Read the model definition and answer for the solid it produces. Units are mm, in the model's axes. A direction names the side the tool comes from. Coordinates: 2 decimals unless noted, no trailing zeros. Loops run counter-clockwise (first coordinate to the right, second up) from the corner with the lowest first, then second, coordinate; pieces in that order, holes last. Notation, with made-up numbers: (26.25, 22) -> (75.25, 22) arc R26 cw to (75.25, 45) -> close; hole circle Ø6 at (-17.75, 0). An arc over 180 degrees is marked (long way). Answer as a JSON object with one key per item and string values. Group by question number.
1) Section A-A, the plane y = -42 is taken. Give the vertices of the cut face in (x, z).
2) Flat-ended cylindrical pins translate along their axes: P1, Ø0.9, axis at x = -29, z = 55.5, coming from the +Y side; P2, Ø7, axis at y = 22, z = -91.5, coming from the -X side; P3, Ø5, axis at x = -17.5, z = -80, coming from the -Y side; P4, Ø3.5, axis at x = -28.5, y = 14, coming from the +Z side. Find the tip coordinate at first contact, or state that the pin passes through.
3) Consider probe 1 along Y at (x, z) = (-28.75, -76.5); probe 2 along Z at (x, y) = (25, -5); probe 3 along Y at (x, z) = (16, 72). Determine where each line is inside the solid, lowest interval first. Write a range as [from, to].
4) Which of the six approach directions +Z, -Z, +X, -X, +Y, -Y give full straight-line access (tool end or side, diameter ignored) to faces 4 (the face through (27.2, 6.6, -110)), 5 (the face through (25.98, -23.707, -115.521)), 6 (the face through (-28.479, 22.121, -73.753))?
5) Section C-C, the plane x = 2.5 is taken. Give the vertices of the cut face in (y, z).
6) Determine the mould class of faces 1 (the face through (1.08, 1.48, 99.88)), 2 (the face through (-29, 28, -96)), 3 (the face through (-23, -1, -113)) for opening direction Z: released by +Z, released by -Z, zero draft, split by the parting line, or undercut.
7) Section D-D, the plane y = -68 is taken. Give the vertices of the cut face in (x, z), plus the area to 3 significant figures.
8) Section B-B, the plane z = 51 is taken. Give the vertices of the cut face in (x, y).
from build123d import *

# Parameters (mm, degrees)
ODGI_CIE_BAZOWE1_DEPTH           = 110
ODGI_CIE_START                   = -40
ODGI_CIE_KRAW_DZI1_OUTLINE_W     = 73
ODGI_CIE_KRAW_DZI1_OUTLINE_H     = 3
ODGI_CIE_KRAW_DZI1_DEPTH         = 80
ODGI_CIE_START_2                 = -23
ODGI_CIE_KRAW_DZI1_2_DEPTH       = 46
WYTNIJ_WYCI_GNI_CIE1_REACH       = 245.019
OTW_R_POD_RUB_M81_D              = 10
OTW_R_POD_RUB_M81_DEPTH          = 10
OTW_R_POD_RUB_M81_TIP            = 3.004303095
SZKIC19_W                        = 25
SZKIC19_H                        = 15
WYTNIJ_WYCI_GNI_CIE2_DEPTH       = 10
ZAOKR_GLENIE1_R                  = 2
WYTNIJ_WYCI_GNI_CIE3_REACH       = 245.019
SZKIC20_R                        = 6.5
WYTNIJ_WYCI_GNI_CIE4_DEPTH       = 157.582246759
ZAOKR_GLENIE2_R                  = 1
SZYK_LINIOWY1_COUNT              = 3
SZYK_LINIOWY1_PITCH              = 70
ZAOKR_GLENIE2_OF_SZYK_LINIOWY1_R = 1
SZKIC22_R                        = 6
WYTNIJ_WYCI_GNI_CIE5_DEPTH       = 244.018517813
ZAOKR_GLENIE3_R                  = 12
SZKIC23_W                        = 30
SZKIC23_H                        = 12
WYPUST2_DEPTH                    = 3
SFAZOWANIE1_SIZE                 = 5
OTW_R_POD_RUB_M52_D              = 5.5


# Read off the part's stored shape, not the designer's step: Odgięcie krawędzi1
# Sheet-metal steps are written as plain solids
with BuildPart() as part:
    # Szkic1 → Odgięcie bazowe1 (new, symmetric)
    with BuildSketch(Plane.XY):
        with BuildLine():
            Line((-30, 18), (-30, 7))
            ThreePointArc((-30, 7), (-27.949747468, 2.050252532), (-23, 0))
            Line((-23, 0), (23, 0))
            ThreePointArc((23, 0), (27.949747468, 2.050252532), (30, 7))
            Line((30, 7), (30, 18))
            Line((30, 18), (27, 18))
            Line((27, 18), (27, 7))
            ThreePointArc((27, 7), (25.828427125, 4.171572875), (23, 3))
            Line((23, 3), (-23, 3))
            ThreePointArc((-23, 3), (-25.828427125, 4.171572875), (-27, 7))
            Line((-27, 7), (-27, 18))
            Line((-27, 18), (-30, 18))
        make_face()
    extrude(amount=ODGI_CIE_BAZOWE1_DEPTH, both=True)



with BuildPart() as body_2:
    # Odgięcie krawędzi1 outline → Odgięcie krawędzi1 (new body)
    with BuildSketch(Plane.YZ.offset(ODGI_CIE_START)):
        with Locations((-40.5, -115.5)):
            Rectangle(ODGI_CIE_KRAW_DZI1_OUTLINE_W, ODGI_CIE_KRAW_DZI1_OUTLINE_H)
    extrude(amount=ODGI_CIE_KRAW_DZI1_DEPTH)


with BuildPart() as part_1:
    add(part.part)

    add(body_2.part)  # Odgi_cie kraw_dzi1 2 merges body 2
    # Odgi_cie kraw_dzi1 2 outline → Odgi_cie kraw_dzi1 2 (add)
    with BuildSketch(Plane.YZ.offset(ODGI_CIE_START_2)):
        with BuildLine():
            Line((-4, -114), (-4, -117))
            ThreePointArc((-4, -117), (0.949747468, -114.949747468), (3, -110))
            Line((3, -110), (0, -110))
            ThreePointArc((0, -110), (-1.171572875, -112.828427125), (-4, -114))
        make_face()
    extrude(amount=ODGI_CIE_KRAW_DZI1_2_DEPTH)

    # Szkic9 → Wytnij-wyciągnięcie1 (cut, up to next)
    with BuildSketch(Plane(origin=(0, 0, -117), x_dir=(-1, 0, 0), z_dir=(0, 0, -1)), mode=Mode.PRIVATE) as wytnij_wyci_gni_cie1_sk1:
        with BuildLine():
            Line((-30.018425021, -20.879449696), (-21.826904579, -26.61521406))
            ThreePointArc((-21.826904579, -26.61521406), (-21.151571657, -30.445217382), (-24.981574979, -31.120550304))
            Line((-24.981574979, -31.120550304), (-33.173095421, -25.38478594))
            ThreePointArc((-33.173095421, -25.38478594), (-33.848428343, -21.554782618), (-30.018425021, -20.879449696))
        make_face()
    wytnij_wyci_gni_cie1_tool1 = extrude(wytnij_wyci_gni_cie1_sk1.sketch, amount=-WYTNIJ_WYCI_GNI_CIE1_REACH, mode=Mode.PRIVATE) & part_1.part
    # Szkic9 → Wytnij-wyciągnięcie1 (cut, up to next)
    with BuildSketch(Plane(origin=(0, 0, -117), x_dir=(-1, 0, 0), z_dir=(0, 0, -1)), mode=Mode.PRIVATE) as wytnij_wyci_gni_cie1_sk2:
        with BuildLine():
            Line((30.018425021, -20.879449696), (21.826904579, -26.61521406))
            ThreePointArc((21.826904579, -26.61521406), (21.151571657, -30.445217382), (24.981574979, -31.120550304))
            Line((24.981574979, -31.120550304), (33.173095421, -25.38478594))
            ThreePointArc((33.173095421, -25.38478594), (33.848428343, -21.554782618), (30.018425021, -20.879449696))
        make_face()
    wytnij_wyci_gni_cie1_tool2 = extrude(wytnij_wyci_gni_cie1_sk2.sketch, amount=-WYTNIJ_WYCI_GNI_CIE1_REACH, mode=Mode.PRIVATE) & part_1.part
    # Szkic9 → Wytnij-wyciągnięcie1 (cut, up to next)
    with BuildSketch(Plane(origin=(0, 0, -117), x_dir=(-1, 0, 0), z_dir=(0, 0, -1)), mode=Mode.PRIVATE) as wytnij_wyci_gni_cie1_sk3:
        with BuildLine():
            Line((-30.018425021, -63.120550304), (-21.826904579, -57.38478594))
            ThreePointArc((-21.826904579, -57.38478594), (-21.151571657, -53.554782618), (-24.981574979, -52.879449696))
            Line((-24.981574979, -52.879449696), (-33.173095421, -58.61521406))
            ThreePointArc((-33.173095421, -58.61521406), (-33.848428343, -62.445217382), (-30.018425021, -63.120550304))
        make_face()
    wytnij_wyci_gni_cie1_tool3 = extrude(wytnij_wyci_gni_cie1_sk3.sketch, amount=-WYTNIJ_WYCI_GNI_CIE1_REACH, mode=Mode.PRIVATE) & part_1.part
    # Szkic9 → Wytnij-wyciągnięcie1 (cut, up to next)
    with BuildSketch(Plane(origin=(0, 0, -117), x_dir=(-1, 0, 0), z_dir=(0, 0, -1)), mode=Mode.PRIVATE) as wytnij_wyci_gni_cie1_sk4:
        with BuildLine():
            Line((30.018425021, -63.120550304), (21.826904579, -57.38478594))
            ThreePointArc((21.826904579, -57.38478594), (21.151571657, -53.554782618), (24.981574979, -52.879449696))
            Line((24.981574979, -52.879449696), (33.173095421, -58.61521406))
            ThreePointArc((33.173095421, -58.61521406), (33.848428343, -62.445217382), (30.018425021, -63.120550304))
        make_face()
    wytnij_wyci_gni_cie1_tool4 = extrude(wytnij_wyci_gni_cie1_sk4.sketch, amount=-WYTNIJ_WYCI_GNI_CIE1_REACH, mode=Mode.PRIVATE) & part_1.part
    add(wytnij_wyci_gni_cie1_tool1.solids().sort_by_distance((27.5, -26, -117))[0], mode=Mode.SUBTRACT)
    add(wytnij_wyci_gni_cie1_tool2.solids().sort_by_distance((-27.5, -26, -117))[0], mode=Mode.SUBTRACT)
    add(wytnij_wyci_gni_cie1_tool3.solids().sort_by_distance((27.5, -58, -117))[0], mode=Mode.SUBTRACT)
    add(wytnij_wyci_gni_cie1_tool4.solids().sort_by_distance((-27.5, -58, -117))[0], mode=Mode.SUBTRACT)

    # Otwór pod śrubę M81
    with Locations(Plane(origin=(0, 3, 0), x_dir=(1, 0, 0), z_dir=(0, 1, 0))):
        with Locations((0, -95), (0, -25)):
            Hole(OTW_R_POD_RUB_M81_D / 2, depth=OTW_R_POD_RUB_M81_DEPTH)
            with Locations((0, 0, -(OTW_R_POD_RUB_M81_DEPTH + OTW_R_POD_RUB_M81_TIP / 2))):  # 118° drill point
                Cone(0, OTW_R_POD_RUB_M81_D / 2, OTW_R_POD_RUB_M81_TIP, mode=Mode.SUBTRACT)

    # Szkic19 → Wytnij-wyciągnięcie2 (cut)
    with BuildSketch(Plane(origin=(0, 3, 0), x_dir=(1, 0, 0), z_dir=(0, 1, 0))):
        with Locations((0, 92.5)):
            Rectangle(SZKIC19_W, SZKIC19_H)
    extrude(amount=-WYTNIJ_WYCI_GNI_CIE2_DEPTH, mode=Mode.SUBTRACT)

    # Zaokrąglenie1
    zaokr_glenie1_edges = [part_1.edges().sort_by_distance(p)[0] for p in [
        (-12.5, 1.5, -85),
        (-12.5, 1.5, -100),
        (12.5, 1.5, -100),
        (12.5, 1.5, -85),
    ]]
    fillet(zaokr_glenie1_edges, radius=ZAOKR_GLENIE1_R)

    # Szkic20 → Wytnij-wyciągnięcie3 (cut, up to next)
    with BuildSketch(Plane(origin=(0, 0, -117), x_dir=(-1, 0, 0), z_dir=(0, 0, -1)), mode=Mode.PRIVATE) as wytnij_wyci_gni_cie3_sk1:
        with Locations(Location((0, -42, 0), (0, 0, 90))):
            Circle(SZKIC20_R)
    wytnij_wyci_gni_cie3_tool1 = extrude(wytnij_wyci_gni_cie3_sk1.sketch, amount=-WYTNIJ_WYCI_GNI_CIE3_REACH, mode=Mode.PRIVATE) & part_1.part
    add(wytnij_wyci_gni_cie3_tool1.solids().sort_by_distance((0, -42, -117))[0], mode=Mode.SUBTRACT)

    # Szkic21 → Wytnij-wyciągnięcie4 (cut, through all)
    with BuildSketch(Plane.ZY.offset(30)):
        Polygon((-55, 18), (-55, 12), (-37, 12), (-37, 15), (-49, 15), (-49, 18), align=None)
    wytnij_wyci_gni_cie4 = extrude(amount=-WYTNIJ_WYCI_GNI_CIE4_DEPTH, mode=Mode.SUBTRACT)

    # Zaokrąglenie2
    zaokr_glenie2_edges = [part_1.edges().sort_by_distance(p)[0] for p in [
        (28.5, 18, -55),
        (28.5, 18, -49),
        (28.5, 15, -49),
        (28.5, 15, -37),
        (28.5, 12, -37),
        (28.5, 12, -55),
        (-28.5, 18, -55),
        (-28.5, 18, -49),
        (-28.5, 15, -49),
        (-28.5, 15, -37),
        (-28.5, 12, -37),
        (-28.5, 12, -55),
    ]]
    fillet(zaokr_glenie2_edges, radius=ZAOKR_GLENIE2_R)

    # Szyk liniowy1: Wytnij-wyciągnięcie4 ×3
    with Locations(*[(0, 0, i * SZYK_LINIOWY1_PITCH) for i in range(1, SZYK_LINIOWY1_COUNT)]):
        add(wytnij_wyci_gni_cie4, mode=Mode.SUBTRACT)

    # Zaokrąglenie2 of Szyk liniowy1
    zaokr_glenie2_of_szyk_liniowy1_edges = [part_1.edges().sort_by_distance(p)[0] for p in [
        (28.5, 18, 15),
        (28.5, 18, 21),
        (28.5, 15, 21),
        (28.5, 15, 33),
        (28.5, 12, 33),
        (28.5, 12, 15),
        (-28.5, 18, 15),
        (-28.5, 18, 21),
        (-28.5, 15, 21),
        (-28.5, 15, 33),
        (-28.5, 12, 33),
        (-28.5, 12, 15),
        (28.5, 18, 85),
        (28.5, 18, 91),
        (28.5, 15, 91),
        (28.5, 15, 103),
        (28.5, 12, 103),
        (28.5, 12, 85),
        (-28.5, 18, 85),
        (-28.5, 18, 91),
        (-28.5, 15, 91),
        (-28.5, 15, 103),
        (-28.5, 12, 103),
        (-28.5, 12, 85),
    ]]
    fillet(zaokr_glenie2_of_szyk_liniowy1_edges, radius=ZAOKR_GLENIE2_OF_SZYK_LINIOWY1_R)

    # Szkic22 → Wytnij-wyciągnięcie5 (cut, through all)
    with BuildSketch(Plane(origin=(0, 0, -117), x_dir=(-1, 0, 0), z_dir=(0, 0, -1))):
        with Locations(Location((-15, -16, 0), (0, 0, 90))):
            Circle(SZKIC22_R)
        with Locations(Location((15, -16, 0), (0, 0, 90))):
            Circle(SZKIC22_R)
        with Locations(Location((-15, -68, 0), (0, 0, 90))):
            Circle(SZKIC22_R)
        with Locations(Location((15, -68, 0), (0, 0, 90))):
            Circle(SZKIC22_R)
    extrude(amount=-WYTNIJ_WYCI_GNI_CIE5_DEPTH, mode=Mode.SUBTRACT)

    # Zaokrąglenie3
    zaokr_glenie3_edges = [part_1.edges().sort_by_distance(p)[0] for p in [
        (40, -4, -115.5),
        (-40, -4, -115.5),
        (-40, -77, -115.5),
        (40, -77, -115.5),
    ]]
    fillet(zaokr_glenie3_edges, radius=ZAOKR_GLENIE3_R)

    # Szkic23 → Wypust2 (add)
    with BuildSketch(Plane.ZY.offset(30)):
        with Locations((-84, 24)):
            Rectangle(SZKIC23_W, SZKIC23_H)
    wypust2 = extrude(amount=-WYPUST2_DEPTH)

    # Lustro2: Wypust2 across plane
    add(wypust2.mirror(Plane(origin=(0, 0, 0), x_dir=(0, 0, 1), z_dir=(1, 0, 0))))

    # Sfazowanie1
    sfazowanie1_edges = [part_1.edges().sort_by_distance(p)[0] for p in [
        (-28.5, 18, -110),
        (28.5, 18, -110),
        (-28.5, 18, 110),
        (-28.5, 30, -99),
        (-28.5, 30, -69),
        (28.5, 18, 110),
        (28.5, 30, -99),
        (28.5, 30, -69),
    ]]
    chamfer(sfazowanie1_edges, length=SFAZOWANIE1_SIZE)

    # Otwór pod śrubę M52 (through all)
    with Locations(Plane.ZY.offset(30)):
        with Locations((-91.5, 22), (-76.5, 22)):
            Hole(OTW_R_POD_RUB_M52_D / 2)


solid = part_1.part
Determined:
{
 "1": {"outline": "(-40, -117) -> (-6.5, -117) -> (-6.5, -114) -> (-40, -114) -> close; (6.5, -117) -> (40, -117) -> (40, -114) -> (6.5, -114) -> close"},
 "2": {"P1": "y = 18", "P2": "x = -30", "P3": "y = 0", "P4": "z = 110"},
 "3": {"probe 1": "[3.01, 19.25], [24.75, 30]", "probe 2": "[-117, -114]", "probe 3": "[0, 3]"},
 "4": {"face 4": "-Z, +X, +Y, -Y", "face 5": "+Z, -Z", "face 6": "+X, -X"},
 "5": {"outline": "(-77, -117) -> (-48, -117) -> (-48, -114) -> (-77, -114) -> close; (-36, -117) -> (-4, -117) arc R7 ccw to (3, -110) -> (3, -100) -> (0, -100) -> (0, -110) arc R4 cw to (-4, -114) -> (-36, -114) -> close; (0, -85) -> (3, -85) -> (3, 20.67) -> (0, 20.67) -> close; (0, 29.33) -> (3, 29.33) -> (3, 90.67) -> (0, 90.67) -> close; (0, 99.33) -> (3, 99.33) -> (3, 110) -> (0, 110) -> close"},
 "6": {"face 1": "undercut", "face 2": "released by -Z", "face 3": "zero draft"},
 "7": {"outline": "(-39.62, -117) -> (-21, -117) -> (-21, -114) -> (-39.62, -114) -> close; (-9, -117) -> (9, -117) -> (9, -114) -> (-9, -114) -> close; (21, -117) -> (39.62, -117) -> (39.62, -114) -> (21, -114) -> close", "area": "166 mm²"},
 "8": {"outline": "(-30, 7) arc R7 ccw to (-23, 0) -> (23, 0) arc R7 ccw to (30, 7) -> (30, 18) -> (27, 18) -> (27, 7) arc R4 cw to (23, 3) -> (-23, 3) arc R4 cw to (-27, 7) -> (-27, 18) -> (-30, 18) -> close"}
}
